Print and shaded views of the part. All mm, measured from the part's lowest x, y and z. A direction names the side the tool comes from. Round coordinates to 2 decimals unless told otherwise and drop trailing zeros. Write each loop counter-clockwise with the first axis right and the second up, starting at its lowest first coordinate (ties: lowest second). Pieces come first, ordered by that corner, then holes. Notation, with made-up numbers: M 16.25,-15 L 25.25,-15 A18 ccw 25.25,-4 Z; hole C 25,80.5 d6. An arc over 180 degrees is marked long. Write item = value, one per line.
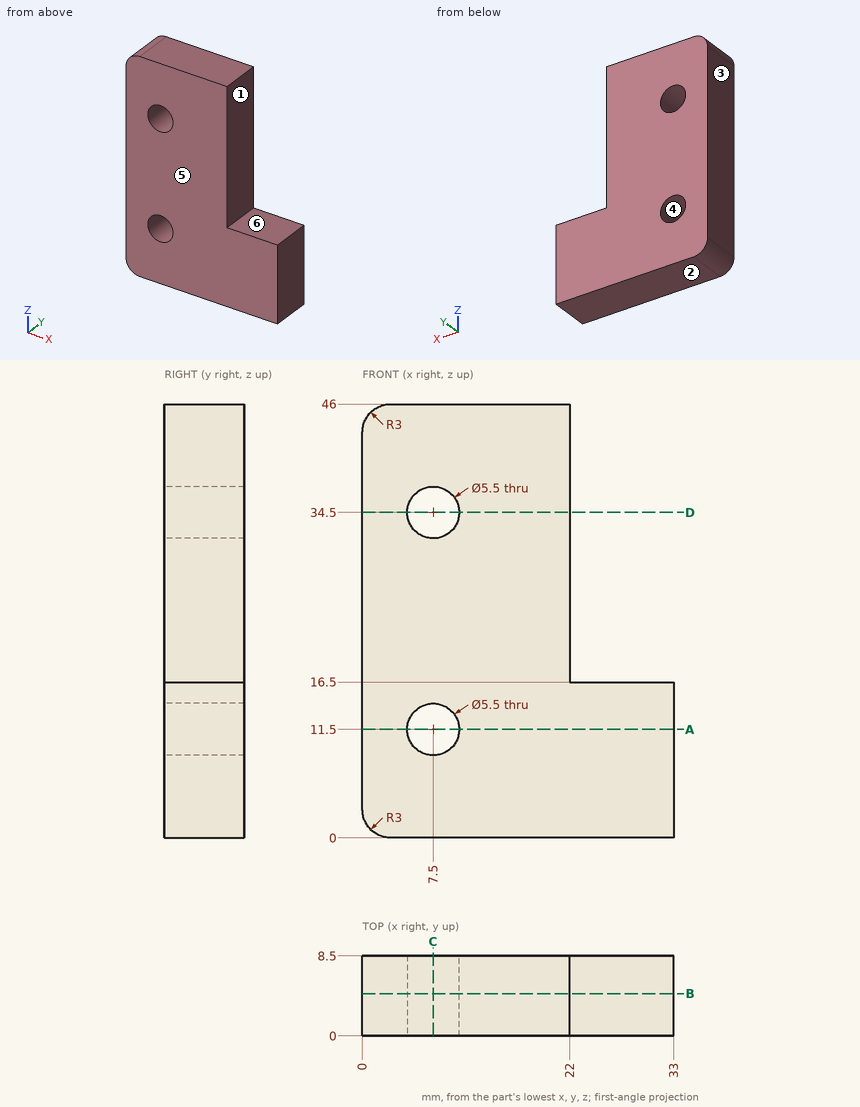
1. Band-saw the part on C-C (x = 7.5). List the corners of the cut face in (y, z), plus the area to 4 significant figures.
Responses:
outline = M 0,0 L 8.5,0 L 8.5,8.75 L 0,8.75 Z; M 0,14.25 L 8.5,14.25 L 8.5,31.75 L 0,31.75 Z; M 0,37.25 L 8.5,37.25 L 8.5,46 L 0,46 Z
area = 297.5 mm²
2. Band-saw the part on B-B (y = 4.5). List the corners of the cut face in (x, z).
Responses:
outline = M 0,3 A3 ccw 3,0 L 33,0 L 33,16.5 L 22,16.5 L 22,46 L 3,46 A3 ccw 0,43 Z; hole C 7.5,11.5 d5.5; hole C 7.5,34.5 d5.5
3. Mould opens along X. For the marked faces 1, 2, 3 and 4 say: pulls with the +X half, pulls with the -X half, needs draft (parallel to the pull), parting line crosses it, or undercut.
Responses:
face_1 = pulls with the +X half
face_2 = needs draft
face_3 = pulls with the -X half
face_4 = undercut
4. Tool access for the marked faces 5 and 6: list every direction of +Z, -Z, +X, -X, +Y, -Y with a clear straight run to the whole face (end or side of a thin tool).
Responses:
face_5 = +Z, -Z, +X, -X, -Y
face_6 = +Z, +X, +Y, -Y
5. Band-saw the part on D-D (z = 34.5). List the corners of the cut face in (x, y), plus the area to 3 significant figures.
Responses:
outline = M 0,0 L 4.75,0 L 4.75,8.5 L 0,8.5 Z; M 10.25,0 L 22,0 L 22,8.5 L 10.25,8.5 Z
area = 140 mm²
6. Probe probe 1 along Z at (x, y) = (7.5, 3); probe 2 along X at (y, z) = (5.5, 34.5); probe 3 along Z at (x, y) = (9, 5.75). List the from-to ranges inside material, lowest first.
Responses:
probe_1 = 0 to 8.75, 14.25 to 31.75, 37.25 to 46
probe_2 = 0 to 4.75, 10.25 to 22
probe_3 = 0 to 9.2, 13.8 to 32.2, 36.8 to 46
7. Flat gauge pins, fed straight in: pin 1 (9 mm diameter, centred on x = 7.5, z = 34.5, fed in from -Y); pin 2 (4 mm diameter, centred on x = 29.5, y = 2.5, fed in from +Z); pin 3 (5 mm diameter, centred on y = 6, z = 23.5, fed in from +X). Where does each tip first touch, or does it go through?
Responses:
pin_1 = 0
pin_2 = 16.5
pin_3 = 22
8. Band-saw the part on A-A (z = 11.5). List the corners of the cut face in (x, y), plus the area to 3 significant figures.
Responses:
outline = M 0,0 L 4.75,0 L 4.75,8.5 L 0,8.5 Z; M 10.25,0 L 33,0 L 33,8.5 L 10.25,8.5 Z
area = 234 mm²
